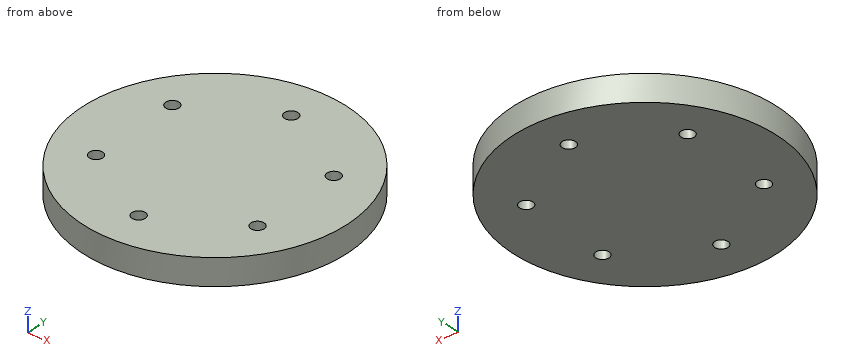
Autodesk Inventor part; units mm, degrees
ref_plane "YZ Plane" through (0, 0, 0) normal (1, 0, 0) x (0, 1, 0)
ref_plane "XZ Plane" through (0, 0, 0) normal (0, 1, 0) x (-1, 0, 0)
ref_plane "XY Plane" through (0, 0, 0) normal (0, 0, 1) x (1, 0, 0)
sketch "Sketch1" plane through (0, 0, 0) normal (0, 0, 1) x (1, 0, 0)
  line L0 (-142.24, 0) -> (142.24, 0)
  line L1 (0, -142.24) -> (0, 142.24)
  circle A0 centre (0, 0) radius 63.5
  circle A1 centre (0, 0) radius 50.8 construction
  circle A2 centre (0, 0) radius 101.6 construction
  dimension "d0" = 101.6
  dimension "d1" = 127
  dimension "d20" = 203.2
extrude "Extrusion1" add sketch "Sketch1" along normal blind 12.7
sketch "Sketch4" plane through (0, 0, 12.7) normal (0, 0, 1) x (1, 0, 0)
  line L0 (-88.9, 0) -> (88.9, 0)
  line L1 (0, -88.9) -> (0, 88.9)
  point P0 (0, 44.45)
  dimension "d21" = 44.45
hole "Hole2" at (0, 44.45, 12.7) direction (0, 0, -1) diameter 6.4008 end through all
pattern_circular "Circular Pattern1" count 6 over 360 about axis through (0, 0, -10) along (0, 0, 1) of "Hole2"
properties part number "wheel hub"
Source: CAD feature listing. Evaluate the final solid. Frame: model axes, mm. Coordinates: 2 decimals unless noted, no trailing zeros. Write each loop counter-clockwise with the first axis right and the second up, starting at its lowest first coordinate (ties: lowest second). Pieces come first, ordered by that corner, then holes. Notation, with made-up numbers: (-26.75, 44) -> (28.25, 44) arc R19 cw to (28.25, 80) -> close; hole circle Ø3 at (18, 55). An arc over 180 degrees is marked (long way). Return JSON: item names as keys, results as strings. Group by question number.
1) Section query B-B, the plane y = -44.45. Return loops of the section in (x, z), plus the area to 3 significant figures.
2) Contact query for flat-ended pins moving along their axis: P1, Ø4, axis at x = 42, z = 6.5, coming from the -Y side; P2, Ø5, axis at y = -28, z = 6, coming from the -X side; P3, Ø2, axis at y = 23.5, z = 9, coming from the -X side. Output: stop coordinate, or through.
3) Section query A-A, the plane x = 0. Return loops of the section in (y, z).
4) Section query C-C, the plane z = 7.75. Return loops of the section in (x, y) (3 decimals), plus the area to 3 significant figures.
5) Ray query, line 1 along X through (y, z) = (-22.5, 3.75); line 2 along Y through (x, z) = (2.5, 4.75); line 3 along X through (y, z) = (22, 12.25). Return the intervals inside material, ascending.
6) Section query D-D, the plane x = 43.5. Return loops of the section in (y, z).
From the geometry:
{
 "1": {"outline": "(-45.35, 0) -> (-3.2, 0) -> (-3.2, 12.7) -> (-45.35, 12.7) -> close; (3.2, 0) -> (45.35, 0) -> (45.35, 12.7) -> (3.2, 12.7) -> close", "area": "1,070 mm²"},
 "2": {"P1": "y = -49.32", "P2": "x = -58.15", "P3": "x = -59.38"},
 "3": {"outline": "(-63.5, 0) -> (-47.65, 0) -> (-47.65, 12.7) -> (-63.5, 12.7) -> close; (-41.25, 0) -> (41.25, 0) -> (41.25, 12.7) -> (-41.25, 12.7) -> close; (47.65, 0) -> (63.5, 0) -> (63.5, 12.7) -> (47.65, 12.7) -> close"},
 "4": {"outline": "circle Ø127 at (0, 0); hole circle Ø6.401 at (-38.495, -22.225); hole circle Ø6.401 at (-38.495, 22.225); hole circle Ø6.401 at (0, -44.45); hole circle Ø6.401 at (0, 44.45); hole circle Ø6.401 at (38.495, -22.225); hole circle Ø6.401 at (38.495, 22.225)", "area": "12,500 mm²"},
 "5": {"line 1": "-59.38 to -41.68, -35.31 to 35.31, 41.68 to 59.38", "line 2": "-63.45 to -46.45, -42.45 to 42.45, 46.45 to 63.45", "line 3": "-59.57 to -41.69, -35.3 to 35.3, 41.69 to 59.57"},
 "6": {"outline": "(-46.26, 0) -> (46.26, 0) -> (46.26, 12.7) -> (-46.26, 12.7) -> close"}
}
